```python
from build123d import *

# Parameters (mm, degrees)
SKETCH1_W                                    = 26
SKETCH1_H                                    = 12.9
BOSS_EXTRUDE1_DEPTH                          = 5.9
SKETCH2_W                                    = 2.95
SKETCH2_H                                    = 2.05
CUT_EXTRUDE1_DEPTH                           = 27
CSK_SLOT_FOR_M2_COUNTERSUNK_FLAT_HEA_2_COUNT = 2
CSK_SLOT_FOR_M2_COUNTERSUNK_FLAT_HEA_2_PITCH = 13
FILLET1_R                                    = 2


with BuildPart() as part:
    # Sketch1 → Boss-Extrude1 (new body)
    with BuildSketch(Plane.XY):
        Rectangle(SKETCH1_W, SKETCH1_H)
    extrude(amount=BOSS_EXTRUDE1_DEPTH)

    # Sketch2 → Cut-Extrude1 (cut, through all)
    with BuildSketch(Plane(origin=(13, 0, 0), x_dir=(0, 0, -1), z_dir=(1, 0, 0))):
        with Locations((-1.475, 5.425)):
            Rectangle(SKETCH2_W, SKETCH2_H)
        with Locations((-1.475, -5.425)):
            Rectangle(SKETCH2_W, SKETCH2_H)
    extrude(amount=-CUT_EXTRUDE1_DEPTH, mode=Mode.SUBTRACT)

    # Sketch3 → CSK SLOT for M2 Countersunk Flat Head Screw1 (revolve, cut)
    with BuildSketch(Plane(origin=(-6.5, 0, 5.9), x_dir=(0, -1, 0), z_dir=(1, 0, 0))):
        Polygon((0, 0), (0, 6.621032743), (1.2, 5.9), (1.2, 5.5), (2.2, 4.5), (2.2, 0), align=None)
    csk_slot_for_m2_countersunk_flat_head_sc = revolve(axis=Axis((-6.5, 0, 12.25), (0, 0, -1)), mode=Mode.SUBTRACT)

    # CSK SLOT for M2 Countersunk Flat Hea 2: CSK SLOT for M2 Countersunk Flat Head Screw1 ×2
    with Locations(*[(i * CSK_SLOT_FOR_M2_COUNTERSUNK_FLAT_HEA_2_PITCH, 0, 0) for i in range(1, CSK_SLOT_FOR_M2_COUNTERSUNK_FLAT_HEA_2_COUNT)]):
        add(csk_slot_for_m2_countersunk_flat_head_sc, mode=Mode.SUBTRACT)

    # Fillet1
    fillet1_edges = [part.edges().sort_by_distance(p)[0] for p in [
        (-13, 0, 5.9),
        (-13, 6.45, 4.425),
        (-13, -6.45, 4.425),
    ]]
    fillet(fillet1_edges, radius=FILLET1_R)


solid = part.part
```
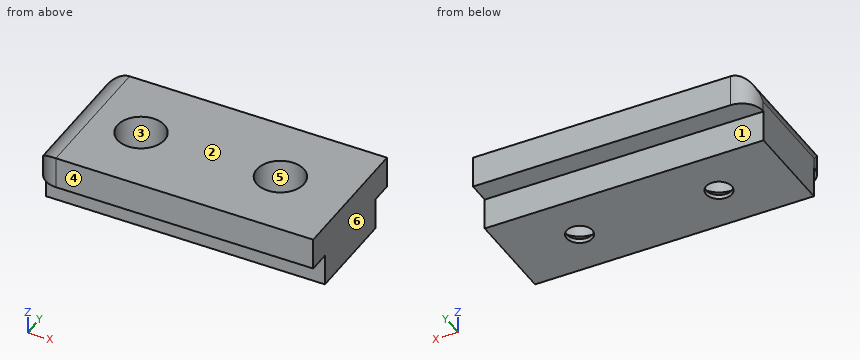
The listing builds one solid part. Answer for the finished solid, in the listing's coordinates (mm). Face numbers are marked on the shaded views. A direction names the side the tool comes from. Round coordinates to 2 decimals unless told otherwise and drop trailing zeros. Write each loop counter-clockwise with the first axis right and the second up, starting at its lowest first coordinate (ties: lowest second). Pieces come first, ordered by that corner, then holes. Notation, with made-up numbers: (-36.5, 78.25) -> (6.5, 78.25) arc R28 ccw to (6.5, 97.25) -> close; hole circle Ø2 at (45, 82). An arc over 180 degrees is marked (long way). Answer as a JSON object with one key per item and string values. Group by question number.
Q1. Section D-D (x = -9) is taken. Write down the section's boundary in (y, z).
Q2. Section C-C (x = 6.5) is taken. Write down the section's boundary in (y, z).
Q3. Each of these flat-tipped pins is pushed along its axis until it touches: pin 1 Ø1 at (x, y) = (4.5, 5.5) entering from -Z; pin 2 Ø1.5 at (x, z) = (0.5, 2) entering from +Y; pin 3 Ø4 at (x, y) = (6.5, 0) entering from +Z. Where does it stop, or does it pass through?
Q4. Section A-A (y = 0) is taken. Write down the section's boundary in (x, z), plus the area to 3 significant figures.
Q5. Which of the six approach directions +Z, -Z, +X, -X, +Y, -Y give full straight-line access (tool end or side, diameter ignored) to the marked faces 1 and 2?
Q6. Straight lines are drawn through the part: line 1 along X through (y, z) = (0, 4.05); line 2 along X through (y, z) = (0, 0.25); line 3 along Y through (x, z) = (6.5, 4.75). For each, find the intervals that lie inside material, in ascending order.
Q7. Section B-B (z = 3.25) is taken. Write down the section's boundary in (x, y).
Q8. Determine the mould class of the marked faces 3, 4, 5 and 6 for opening direction Y: pulls with the +Y half, pulls with the -Y half, needs draft (parallel to the pull), parting line crosses it, or undercut.
Check values:
{
 "1": {"outline": "(-6.45, 2.95) -> (-4.4, 2.95) -> (-4.4, 0) -> (4.4, 0) -> (4.4, 2.95) -> (6.45, 2.95) -> (6.45, 5.9) -> (-6.45, 5.9) -> close"},
 "2": {"outline": "(-6.45, 2.95) -> (-4.4, 2.95) -> (-4.4, 0) -> (-1.2, 0) -> (-1.2, 0.4) -> (-2.2, 1.4) -> (-2.2, 5.9) -> (-6.45, 5.9) -> close; (1.2, 0) -> (4.4, 0) -> (4.4, 2.95) -> (6.45, 2.95) -> (6.45, 5.9) -> (2.2, 5.9) -> (2.2, 1.4) -> (1.2, 0.4) -> close"},
 "3": {"pin 1": "z = 2.95", "pin 2": "y = 4.4", "pin 3": "z = 1.2"},
 "4": {"outline": "(-13, 0) -> (-7.7, 0) -> (-7.7, 0.4) -> (-8.7, 1.4) -> (-8.7, 5.9) -> (-11, 5.9) arc R2 ccw to (-13, 3.9) -> close; (-5.3, 0) -> (5.3, 0) -> (5.3, 0.4) -> (4.3, 1.4) -> (4.3, 5.9) -> (-4.3, 5.9) -> (-4.3, 1.4) -> (-5.3, 0.4) -> close; (7.7, 0) -> (13, 0) -> (13, 5.9) -> (8.7, 5.9) -> (8.7, 1.4) -> (7.7, 0.4) -> close", "area": "104 mm^2"},
 "5": {"face 1": "-Z, +X, -X, +Y", "face 2": "+Z, +X, -X, +Y, -Y"},
 "6": {"line 1": "-12.99 to -8.7, -4.3 to 4.3, 8.7 to 13", "line 2": "-13 to -7.7, -5.3 to 5.3, 7.7 to 13", "line 3": "-6.45 to -2.2, 2.2 to 6.45"},
 "7": {"outline": "(-13, -4.45) arc R2 ccw to (-11, -6.45) -> (13, -6.45) -> (13, 6.45) -> (-11, 6.45) arc R2 ccw to (-13, 4.45) -> close; hole circle Ø4.4 at (-6.5, 0); hole circle Ø4.4 at (6.5, 0)"},
 "8": {"face 3": "undercut", "face 4": "pulls with the -Y half", "face 5": "undercut", "face 6": "needs draft"}
}
